Work out the finished part from the listing and answer in its coordinate system (mm). A direction names the side the tool comes from. Give positions to 0.01 mm unless a question says otherwise; leave off trailing zeros. Order: outer loops, then holes, each group sorted by start corner. A loop starts at its lowest first (then second) coordinate and runs counter-clockwise, first axis right, second up. Notation, with made-up numbers: (34, -9.75) -> (83, -9.75) arc R22 cw to (83, 19.25) -> close; hole circle Ø1 at (89, 80). An arc over 180 degrees is marked (long way). Use a Markdown table: item, result. Add a question column.
```python
from build123d import *

# Parameters (mm, degrees)
F1_DEPTH = 25
F3_R     = 8.940087
F4_DEPTH = 50
F5_R     = 10


with BuildPart() as f1:
    # F0 (on Top) → F1 (new body)
    with BuildSketch(Plane.XY):
        with BuildLine():
            ThreePointArc((76, 0), (0, -76), (-76, 0))
            Line((-76, 0), (-106, 0))
            Line((-106, 0), (-106, -2))
            Line((-106, -2), (-77.974355, -2))
            ThreePointArc((-77.974355, -2), (0, -78), (77.974355, -2))
            Line((77.974355, -2), (106, -2))
            Line((106, -2), (106, 0))
            Line((106, 0), (76, 0))
        make_face()
    extrude(amount=F1_DEPTH)

    # F3 (on offset) → F4 (join)
    with BuildSketch(Plane.XZ.offset(76.3)):
        with Locations((0, 12.596033)):
            Circle(F3_R)
    extrude(amount=F4_DEPTH)

    # F5
    f5_edges = [f1.edges().sort_by_distance(p)[0] for p in [
        (106, -1, 25),
        (106, -1, 0),
        (-106, -1, 25),
        (-106, -1, 0),
    ]]
    fillet(f5_edges, radius=F5_R)


solid = f1.part
```
1) The part is cut by section D-D, the plane y = -89.5. Determine the outline of the cut face in (x, z).
2) The part is cut by section A-A, the plane x = 0. Determine the outline of the cut face in (y, z), then the cut area to 3 significant figures.
3) Straight lines are drawn through the part: line 1 (Y direction, x = 1, z = 10.5); line 2 (X direction, y = -41.5, z = 1.5); line 3 (X direction, y = -38, z = 10). For each, find the intervals that lie inside material, in ascending order.
4) Which of the six approach directions +Z, -Z, +X, -X, +Y, -Y give full straight-line access (tool end or side, diameter ignored) to faces 5 (the flat face through (-0.4, -76.4, 0)), 6 (the flat face through (-92, -2, 12)), 7 (the cylindrical face through (8.527, -101.551, 15.281)), 8 (the flat face through (92, -2, 12))?
5) Determine the mould class of faces 1 (the flat face through (-91, 0, 12)), 2 (the cylindrical face through (1.67, -75.98, 12.32)), 3 (the cylindrical face through (-1.69, -77.98, 23.44)), 4 (the cylindrical face through (102.99, -0.99, 2.85)) for opening direction X: released by +X, released by -X, zero draft, split by the parting line, or undercut.
6) The part is cut by section C-C, the plane z = 17.5. Determine the outline of the cut face in (x, y), then the cut area to 3 significant figures.
7) Flat-ended cylindrical pins translate along their axes: pin 1 (1.5 mm diameter, centred on x = -55, z = 9.5, fed in from -Y); pin 2 (3 mm diameter, centred on x = 57, z = 4.5, fed in from +Y); pin 3 (6 mm diameter, centred on x = 2.5, z = 16.5, fed in from +Y). Find the tip coordinate at first contact, or state that the pin passes through.
A:
| question | item | result |
|---|---|---|
| 1 | outline | circle Ø17.88 at (0, 12.6) |
| 2 | outline | (-126.3, 3.66) -> (-78, 3.66) -> (-78, 0) -> (-76, 0) -> (-76, 25) -> (-78, 25) -> (-78, 21.54) -> (-126.3, 21.54) -> close |
| 2 | area | 914 mm^2 |
| 3 | line 1 | -126.3 to -75.99 |
| 3 | line 2 | -66.04 to -63.67, 63.67 to 66.04 |
| 3 | line 3 | -68.12 to -65.82, 65.82 to 68.12 |
| 4 | face 5 | -Z, +X, -X, +Y, -Y |
| 4 | face 6 | +Z, -Z, -X, -Y |
| 4 | face 7 | -Y |
| 4 | face 8 | +Z, -Z, +X, -Y |
| 5 | face 1 | zero draft |
| 5 | face 2 | undercut |
| 5 | face 3 | split by the parting line |
| 5 | face 4 | released by +X |
| 6 | outline | (-105.68, -2) -> (-77.97, -2) arc R78 ccw to (-7.48, -77.64) -> (-7.48, -126.3) -> (7.48, -126.3) -> (7.48, -77.64) arc R78 ccw to (77.97, -2) -> (105.68, -2) -> (105.68, 0) -> (76, 0) arc R76 cw to (-76, 0) -> (-105.68, 0) -> close |
| 6 | area | 1,320 mm^2 |
| 7 | pin 1 | y = -56.04 |
| 7 | pin 2 | y = -48.52 |
| 7 | pin 3 | y = -75.8 |
